```python
from build123d import *

# Parameters (mm, degrees)
SKETCH2_R          = 3.175
CUT_EXTRUDE1_DEPTH = 72.584302274


with BuildPart() as part:
    # Sketch1 → Revolve1 (revolve)
    with BuildSketch(Plane.XY, mode=Mode.PRIVATE) as revolve1_sk:
        with BuildLine():
            Line((0, 0), (3.81, 0))
            Line((3.81, 0), (3.81, 50.546))
            Line((3.81, 50.546), (3.530377137, 50.546))
            ThreePointArc((3.530377137, 50.546), (1.963328877, 49.2125), (0.396280616, 50.546))
            Line((0.396280616, 50.546), (0, 50.546))
            Line((0, 50.546), (0, 0))
        make_face()
    revolve(revolve1_sk.sketch.rotate(Axis((0, 0, 0), (1, 0, 0)), 90), axis=Axis((0, 0, 0), (1, 0, 0)))

    # Sketch2 → Cut-Extrude1 (cut, through all)
    with BuildSketch(Plane(origin=(3.81, 0, 0), x_dir=(0, 0, -1), z_dir=(1, 0, 0))):
        with BuildLine():
            Line((-38.511581654, 21.479742361), (-10.413064573, 5.807861807))
            ThreePointArc((-10.413064573, 5.807861807), (-7.397844739, 9.350671943), (-3.256370105, 11.46992704))
            Line((-3.256370105, 11.46992704), (-12.04332906, 42.420272023))
            ThreePointArc((-12.04332906, 42.420272023), (-27.360120522, 34.582438584), (-38.511581654, 21.479742361))
        make_face()
        with BuildLine():
            Line((21.479742361, 38.511581654), (5.807861807, 10.413064573))
            ThreePointArc((5.807861807, 10.413064573), (9.350671943, 7.397844739), (11.46992704, 3.256370105))
            Line((11.46992704, 3.256370105), (42.420272023, 12.04332906))
            ThreePointArc((42.420272023, 12.04332906), (34.582438584, 27.360120522), (21.479742361, 38.511581654))
        make_face()
        with BuildLine():
            Line((38.511581654, -21.479742361), (10.413064573, -5.807861807))
            ThreePointArc((10.413064573, -5.807861807), (7.397844739, -9.350671943), (3.256370105, -11.46992704))
            Line((3.256370105, -11.46992704), (12.04332906, -42.420272023))
            ThreePointArc((12.04332906, -42.420272023), (27.360120522, -34.582438584), (38.511581654, -21.479742361))
        make_face()
        with BuildLine():
            Line((-21.479742361, -38.511581654), (-5.807861807, -10.413064573))
            ThreePointArc((-5.807861807, -10.413064573), (-9.350671943, -7.397844739), (-11.46992704, -3.256370105))
            Line((-11.46992704, -3.256370105), (-42.420272023, -12.04332906))
            ThreePointArc((-42.420272023, -12.04332906), (-34.582438584, -27.360120522), (-21.479742361, -38.511581654))
        make_face()
        Circle(SKETCH2_R)
    extrude(amount=-CUT_EXTRUDE1_DEPTH, mode=Mode.SUBTRACT)


solid = part.part
```
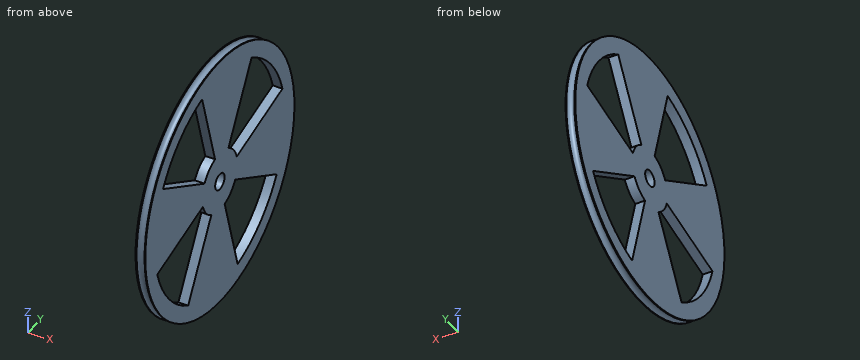
Read the model definition and answer for the solid it produces. Units are mm, in the model's axes. Give positions to 0.01 mm unless a question says otherwise; leave off trailing zeros. Order: outer loops, then holes, each group sorted by start corner. A loop starts at its lowest first (then second) coordinate and runs counter-clockwise, first axis right, second up. Notation, with made-up numbers: (13.5, 30) -> (25.5, 30) arc R18 cw to (25.5, 57) -> close; hole circle Ø6 at (68, 68.5). An arc over 180 degrees is marked (long way). One line per item, written item: value. Start each with the question number.
(1) The part is cut by section D-D (z = -14.5). State how many separate pieces and enclosed holes the cut face has, and give its area (3 significant figures).
(2) Straight lines are drawn through the part: L1, parallel to Z at x = 3.1, y = 29; L2, parallel to Y at x = 3.65, z = -12.5; L3, parallel to Z at x = 0.9, y = 30.5. For each, find the intervals that lie inside material, in ascending order.
(3) Flat-ended cylindrical pins translate along their axes: P1, Ø1.5, axis at x = 2.5, y = -36.5, coming from the +Z side; P2, Ø2, axis at x = 3, z = -39.5, coming from the -Y side. Find the tip coordinate at first contact, or state that the pin passes through.
(4) The part is cut by section C-C (x = 1.65). Determine the outline of the cut face in (y, z) (3 decimals).
Taken from the geometry:
1. separate pieces: 3
1. enclosed holes: 0
1. area: 151 mm^2
2. L1: -40.35 to -33.22, -16.17 to 8.23, 33.22 to 40.35
2. L2: -48.98 to -42.29, -6.97 to 3.55, 22.41 to 48.98
2. L3: -39.14 to -31.85, -17.01 to 8.66, 31.85 to 39.14
3. P1: z = 34.2
3. P2: y = -32.57
4. outline: circle Ø98.487 at (0, 0); hole (-42.42, -12.043) arc R44.097 ccw to (-21.48, -38.512) -> (-5.808, -10.413) arc R11.923 cw to (-11.47, -3.256) -> close; hole (-38.512, 21.48) -> (-10.413, 5.808) arc R11.923 cw to (-3.256, 11.47) -> (-12.043, 42.42) arc R44.097 ccw to start; hole circle Ø6.35 at (0, 0); hole (3.256, -11.47) -> (12.043, -42.42) arc R44.097 ccw to (38.512, -21.48) -> (10.413, -5.808) arc R11.923 cw to start; hole (5.808, 10.413) arc R11.923 cw to (11.47, 3.256) -> (42.42, 12.043) arc R44.097 ccw to (21.48, 38.512) -> close
